```python
from build123d import *

# Parameters (mm, degrees)
BOSS_EXTRUDE1_DEPTH               = 12.7
F_1_4_CLEARANCE_HOLE1_D           = 6.7564
F_1_4_CLEARANCE_HOLE1_CSINK_D     = 8.0264
F_1_4_CLEARANCE_HOLE1_CSINK_ANGLE = 90


with BuildPart() as part:
    # Sketch1 → Boss-Extrude1 (new, symmetric)
    with BuildSketch(Plane.XY):
        with BuildLine():
            Line((-50.700684167, 47.625), (-66.575684167, 47.625))
            Line((-66.575684167, 47.625), (-66.575684167, 34.925))
            Line((-66.575684167, 34.925), (-53.577595831, 34.925))
            ThreePointArc((-53.577595831, 34.925), (0, -5.08), (53.577595831, 34.925))
            Line((53.577595831, 34.925), (66.575684167, 34.925))
            Line((66.575684167, 34.925), (66.575684167, 47.625))
            Line((66.575684167, 47.625), (50.700684167, 47.625))
            ThreePointArc((50.700684167, 47.625), (0, 0), (-50.700684167, 47.625))
        make_face()
    extrude(amount=BOSS_EXTRUDE1_DEPTH, both=True)

    # 1/4 Clearance Hole1 (through all)
    with Locations(Plane(origin=(0, 34.925, 0), x_dir=(-1, 0, 0), z_dir=(0, -1, 0))):
        with Locations((60.076639999, 0), (-60.076639999, 0)):
            CounterSinkHole(F_1_4_CLEARANCE_HOLE1_D / 2, F_1_4_CLEARANCE_HOLE1_CSINK_D / 2, counter_sink_angle=F_1_4_CLEARANCE_HOLE1_CSINK_ANGLE)


solid = part.part
```
Check sheet for the modelled part. Datum: model origin and axes. Units: mm. A direction names the side the tool comes from. Give positions to 0.01 mm unless a question says otherwise; leave off trailing zeros. Loops run counter-clockwise (first coordinate to the right, second up) from the corner with the lowest first, then second, coordinate; pieces in that order, holes last. Notation, with made-up numbers: M -32.75,-2 L -23.75,-2 A23 cw -23.75,29 Z; hole C 62,-10.75 d4. An arc over 180 degrees is marked long. Answer in a Markdown table with one row per item.
1) Mould release check, pull along Z, two halves, no side actions. Record for faces 4 (the face through (63.3, 41.68, -1.01)), 5 (the face through (1.07, 0.01, 0.18)), 6 (the face through (5, 0, -12.7)): released by +Z, released by -Z, zero draft, split by the parting line, or undercut.
Solutions:
| item | result |
|---|---|
| face 4 | undercut |
| face 5 | zero draft |
| face 6 | released by -Z |
2) Cross-section at A-A (z = 0). Enter the section's corners in (x, y) (3 decimals).
Solutions:
| item | result |
|---|---|
| outline | M -66.576,34.925 L -64.09,34.925 L -63.455,35.56 L -63.455,47.625 L -66.576,47.625 Z; M -56.698,35.56 L -56.063,34.925 L -53.578,34.925 A55.88 ccw 53.578,34.925 L 56.063,34.925 L 56.698,35.56 L 56.698,47.625 L 50.701,47.625 A50.8 cw -50.701,47.625 L -56.698,47.625 Z; M 63.455,35.56 L 64.09,34.925 L 66.576,34.925 L 66.576,47.625 L 63.455,47.625 Z |
3) Tool access check on faces 1 (the face through (57, 47.625, 3)), 2 (the face through (57, 34.925, 3)), 3 (the face through (-63, 34.925, 3)). Record the directions out of +Z, -Z, +X, -X, +Y, -Y that give a thin tool (end or side, any length) a straight path to the whole face; none if there is none.
Solutions:
| item | result |
|---|---|
| face 1 | +Z, -Z, +X, -X, +Y |
| face 2 | +Z, -Z, +X, -Y |
| face 3 | +Z, -Z, -X, -Y |
4) Depth check by flat-ended pin: pin 1 (10 mm diameter, centred on x = -21.5, z = -5, fed in from -Y); pin 2 (14.5 mm diameter, centred on x = -61.5, z = -1, fed in from -Y) (3 decimals); pin 3 (12 mm diameter, centred on x = 11, z = -5, fed in from -Y). Enter the tip coordinate at first touch or a pass-through.
Solutions:
| item | result |
|---|---|
| pin 1 | stops at y = -2.59 |
| pin 2 | stops at y = 34.925 |
| pin 3 | stops at y = -4.86 |
5) Cross-section at B-B (y = 39). Enter the section's corners in (x, z).
Solutions:
| item | result |
|---|---|
| outline | M -66.58,-12.7 L -49.41,-12.7 L -49.41,12.7 L -66.58,12.7 Z; M 49.41,-12.7 L 66.58,-12.7 L 66.58,12.7 L 49.41,12.7 Z; hole C -60.08,0 d6.76; hole C 60.08,0 d6.76 |
6) Cross-section at D-D (z = 6.25). Enter the section's corners in (x, y) (3 decimals), plus the area to 3 significant figures.
Solutions:
| item | result |
|---|---|
| outline | M -66.576,34.925 L -53.578,34.925 A55.88 ccw 53.578,34.925 L 66.576,34.925 L 66.576,47.625 L 50.701,47.625 A50.8 cw -50.701,47.625 L -66.576,47.625 Z |
| area | 1,110 mm^2 |
7) Thickness scan on line 1 (Y direction, x = 1.5, z = -4.5); line 2 (X direction, y = 4, z = 6); line 3 (X direction, y = 31.5, z = -10). Record the ranges inside material, lowest first.
Solutions:
| item | result |
|---|---|
| line 1 | y = -5.06 to 0.02 |
| line 2 | x = -30.53 to -19.76, 19.76 to 30.53 |
| line 3 | x = -52.44 to -46.99, 46.99 to 52.44 |
8) Cross-section at C-C (y = 11). Enter the section's corners in (x, z).
Solutions:
| item | result |
|---|---|
| outline | M -39.22,-12.7 L -31.57,-12.7 L -31.57,12.7 L -39.22,12.7 Z; M 31.57,-12.7 L 39.22,-12.7 L 39.22,12.7 L 31.57,12.7 Z |
